Geometry check sheet. Reference: the model listing, model coordinates, mm. A direction names the side the tool comes from. Give positions to 0.01 mm unless a question says otherwise; leave off trailing zeros. Loops run counter-clockwise (first coordinate to the right, second up) from the corner with the lowest first, then second, coordinate; pieces in that order, holes last. Notation, with made-up numbers: (62, 42) -> (121, 42) arc R28 ccw to (121, 65) -> close; hole circle Ø9 at (85.5, 6.25). An arc over 180 degrees is marked (long way). Write each question's results on one line, items separated by ' | '. Start each with the question number.
1) Set-up check for faces 1 (the face through (3, 0, 5.4)), 2 (the face through (0, 133, 0)): record each of +Z, -Z, +X, -X, +Y, -Y from which the full face is reachable in a straight line by a thin tool's end or side.
2) Sectioned sample at D-D on x = 9.5. Record the cut outline in (y, z).
3) Scan lines: line 1 (Y direction, x = 9, z = -4.25); line 2 (X direction, y = 26, z = 9.25); line 3 (Z direction, x = -3.5, y = 77). Record each from-to range of solid material in increasing order. Write a range as from..to.
4) Depth check by flat-ended pin: pin 1 (1 mm diameter, centred on y = 9.5, z = 3.5, fed in from -X); pin 2 (10 mm diameter, centred on x = -6, z = 10, fed in from -Y); pin 3 (8 mm diameter, centred on x = 7.5, y = 27.5, fed in from +Z). Enter the tip coordinate at first touch or a pass-through.
5) Sectioned sample at A-A on x = 0. Record the cut outline in (y, z), then the cut area to 3 significant figures.
6) Sectioned sample at B-B on z = 0. Record the cut outline in (x, y).
7) Sectioned sample at C-C on y = 73.5. Record the cut outline in (x, z).
```python
from build123d import *

# Parameters (mm, degrees)
SKETCH1_R           = 12.5
BOSS_EXTRUDE1_DEPTH = 133
SKETCH2_R           = 10
BOSS_EXTRUDE2_DEPTH = 20


# Read off the part's stored shape, not the designer's step: M12x1.5 Machine Threads Stud1
with BuildPart() as part:
    # Sketch1 → Boss-Extrude1 (new body)
    with BuildSketch(Plane(origin=(0, 0, 0), x_dir=(1, 0, 0), z_dir=(0, 1, 0))):
        with Locations(Location((0, 0, 0), (0, 0, 270))):
            Circle(SKETCH1_R)
    extrude(amount=BOSS_EXTRUDE1_DEPTH)

    # Sketch2 → Boss-Extrude2 (add)
    with BuildSketch(Plane.XZ):
        with Locations(Location((0, 0, 0), (0, 0, 270))):
            Circle(SKETCH2_R)
    extrude(amount=BOSS_EXTRUDE2_DEPTH)

    # M12x1.5 Machine Threads Stud1 outline → M12x1.5 Machine Threads Stud1 (revolve, cut)
    with BuildSketch(Plane.XY):
        Polygon((10, 0), (6, 0), (6, -19.172), (5.172, -20), (10, -20), align=None)
    revolve(axis=Axis((0, 0, 0), (0, 1, 0)), mode=Mode.SUBTRACT)


solid = part.part
```
Result:
1) face 1: -Y | face 2: +Z, -Z, +X, -X, +Y
2) outline: (0, -8.12) -> (133, -8.12) -> (133, 8.12) -> (0, 8.12) -> close
3) line 1: 0..133 | line 2: -8.41..8.41 | line 3: -12..12
4) pin 1: x = -12.13 | pin 2: y = 0 | pin 3: z = 12
5) outline: (-20, -5.17) -> (-19.17, -6) -> (0, -6) -> (0, -12.5) -> (133, -12.5) -> (133, 12.5) -> (0, 12.5) -> (0, 6) -> (-19.17, 6) -> (-20, 5.17) -> close | area: 3,560 mm^2
6) outline: (-12.5, 0) -> (-6, 0) -> (-6, -19.17) -> (-5.17, -20) -> (5.17, -20) -> (6, -19.17) -> (6, 0) -> (12.5, 0) -> (12.5, 133) -> (-12.5, 133) -> close
7) outline: circle Ø25 at (0, 0)
